```python
from build123d import *

# Parameters (mm, degrees)
BOSS_EXTRUDE1_DEPTH = 14.2
SKETCH2_R           = 2.25
CUT_EXTRUDE1_DEPTH  = 15.2
SKETCH3_R           = 3.95
CUT_EXTRUDE2_DEPTH  = 10
SKETCH4_OUTSIDE_W   = 21.704
SKETCH4_OUTSIDE_H   = 20.312
SKETCH4_OUTSIDE_R   = 3.325
CUT_EXTRUDE3_DEPTH  = 10
CUT_EXTRUDE3_TAPER  = 15
SKETCH5_OUTSIDE_W   = 16.344
SKETCH5_OUTSIDE_H   = 14.952
SKETCH5_OUTSIDE_R   = 4.5
CUT_EXTRUDE4_DEPTH  = 1.2
SKETCH6_OUTSIDE_W   = 50.986
SKETCH6_OUTSIDE_H   = 49.594
SKETCH6_OUTSIDE_R   = 4.5
CUT_EXTRUDE5_DEPTH  = 10
CUT_EXTRUDE5_TAPER  = 60


with BuildPart() as part:
    # Sketch1 → Boss-Extrude1 (new body)
    with BuildSketch(Plane(origin=(0, 0, 0), x_dir=(1, 0, 0), z_dir=(0, 1, 0))):
        Polygon((-2.598076211, -4.5), (2.598076211, -4.5), (5.196152423, 0), (2.598076211, 4.5), (-2.598076211, 4.5), (-5.196152423, 0), align=None)
    extrude(amount=BOSS_EXTRUDE1_DEPTH)

    # Sketch2 → Cut-Extrude1 (cut, through all)
    with BuildSketch(Plane(origin=(0, 14.2, 0), x_dir=(1, 0, 0), z_dir=(0, 1, 0))):
        Circle(SKETCH2_R)
    extrude(amount=-CUT_EXTRUDE1_DEPTH, mode=Mode.SUBTRACT)

    # Sketch3 → Cut-Extrude2 (cut)
    with BuildSketch(Plane.XZ):
        Circle(SKETCH3_R)
    extrude(amount=-CUT_EXTRUDE2_DEPTH, mode=Mode.SUBTRACT)

    # Sketch4 outside → Cut-Extrude3 (cut)
    with BuildSketch(Plane(origin=(0, 14.2, 0), x_dir=(1, 0, 0), z_dir=(0, 1, 0))):
        Rectangle(SKETCH4_OUTSIDE_W, SKETCH4_OUTSIDE_H)
        Circle(SKETCH4_OUTSIDE_R, mode=Mode.SUBTRACT)
    extrude(amount=-CUT_EXTRUDE3_DEPTH, taper=CUT_EXTRUDE3_TAPER, mode=Mode.SUBTRACT)

    # Sketch5 outside → Cut-Extrude4 (cut)
    with BuildSketch(Plane.XZ):
        Rectangle(SKETCH5_OUTSIDE_W, SKETCH5_OUTSIDE_H)
        Circle(SKETCH5_OUTSIDE_R, mode=Mode.SUBTRACT)
    extrude(amount=-CUT_EXTRUDE4_DEPTH, mode=Mode.SUBTRACT)

    # Sketch6 outside → Cut-Extrude5 (cut)
    with BuildSketch(Plane.XZ.offset(-1.2)):
        Rectangle(SKETCH6_OUTSIDE_W, SKETCH6_OUTSIDE_H)
        Circle(SKETCH6_OUTSIDE_R, mode=Mode.SUBTRACT)
    extrude(amount=-CUT_EXTRUDE5_DEPTH, taper=CUT_EXTRUDE5_TAPER, mode=Mode.SUBTRACT)


solid = part.part
```
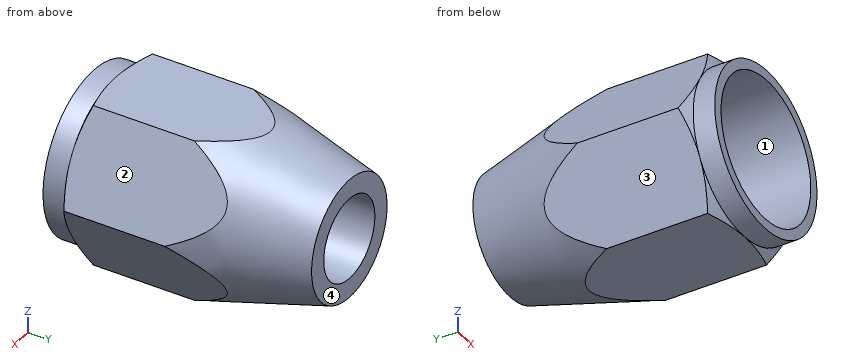
Can you work these out from the model? Positions are in its coordinate system, mm. Face numbers are marked on the shaded views. A direction names the side the tool comes from. Round coordinates to 2 decimals unless told otherwise and drop trailing zeros. Loops run counter-clockwise (first coordinate to the right, second up) from the corner with the lowest first, then second, coordinate; pieces in that order, holes last. Notation, with made-up numbers: M -38.75,41.5 L -17.75,41.5 A34 cw -17.75,78.5 Z; hole C 74,-24.5 d1. An arc over 180 degrees is marked long. Answer in a Markdown table with one row per item.
1. I'm going to push flat-ended pins straight in: pin 1 Ø2.5 at (x, z) = (0, -1.5) entering from -Y; pin 2 Ø2 at (x, y) = (2, 11.5) entering from +Z; pin 3 Ø5 at (x, z) = (0, 0) entering from +Y. Where does each tip first touch, or does it pass through?
Established:
| item | result |
|---|---|
| pin 1 | y = 10 |
| pin 2 | z = 4.04 |
| pin 3 | y = 14.2 |
2. Thinking about a two-plate mould opening in Y: for the marked faces 3 and 4, which applies, pulls with the +Y half, pulls with the -Y half, needs draft (parallel to the pull), parting line crosses it, or undercut?
Established:
| item | result |
|---|---|
| face 3 | needs draft |
| face 4 | pulls with the +Y half |
3. On a 3-axis mill with a long thin cutter (end or side, diameter ignored), from which of +Z, -Z, +X, -X, +Y, -Y can I reach the whole of each face in a straight line? I mean the marked faces 1 and 2. Say none if no direction works.
Established:
| item | result |
|---|---|
| face 1 | -Y |
| face 2 | +Z, +X, +Y, -Y |
4. If we section it at B-B, the plane y = 8: Please give me the cut outline in (x, z), plus the area to 3 significant figures.
Established:
| item | result |
|---|---|
| outline | M -4.97,-0.39 L -2.82,-4.11 A4.99 ccw -2.15,-4.5 L 2.15,-4.5 A4.99 ccw 2.82,-4.11 L 4.97,-0.39 A4.99 ccw 4.97,0.39 L 2.82,4.11 A4.99 ccw 2.15,4.5 L -2.15,4.5 A4.99 ccw -2.82,4.11 L -4.97,0.39 A4.99 ccw Z; hole C 0,0 d7.9 |
| area | 20.7 mm² |
5. If we section it at C-C, the plane y = 9.5: Please give me the cut outline in (x, z).
Established:
| item | result |
|---|---|
| outline | M -4.33,-1.49 L -3.46,-3.01 A4.58 ccw -0.88,-4.5 L 0.88,-4.5 A4.58 ccw 3.46,-3.01 L 4.33,-1.49 A4.58 ccw 4.33,1.49 L 3.46,3.01 A4.58 ccw 0.88,4.5 L -0.88,4.5 A4.58 ccw -3.46,3.01 L -4.33,1.49 A4.58 ccw Z; hole C 0,0 d7.9 |
6. Please list where these lines run through material, in increasing order: line 1 (Z direction, x = 0, y = 7); line 2 (X direction, y = 5.5, z = -2.5); line 3 (Y direction, x = -2.75, z = -1). Write a range as from..to.
Established:
| item | result |
|---|---|
| line 1 | -4.5..-3.95, 3.95..4.5 |
| line 2 | -3.75..-3.06, 3.06..3.75 |
| line 3 | 10..14.2 |
7. If we section it at A-A, the plane y = 3.5: Please give me the cut outline in (x, z).
Established:
| item | result |
|---|---|
| outline | M -5.2,0 L -2.6,-4.5 L 2.6,-4.5 L 5.2,0 L 2.6,4.5 L -2.6,4.5 Z; hole C 0,0 d7.9 |
